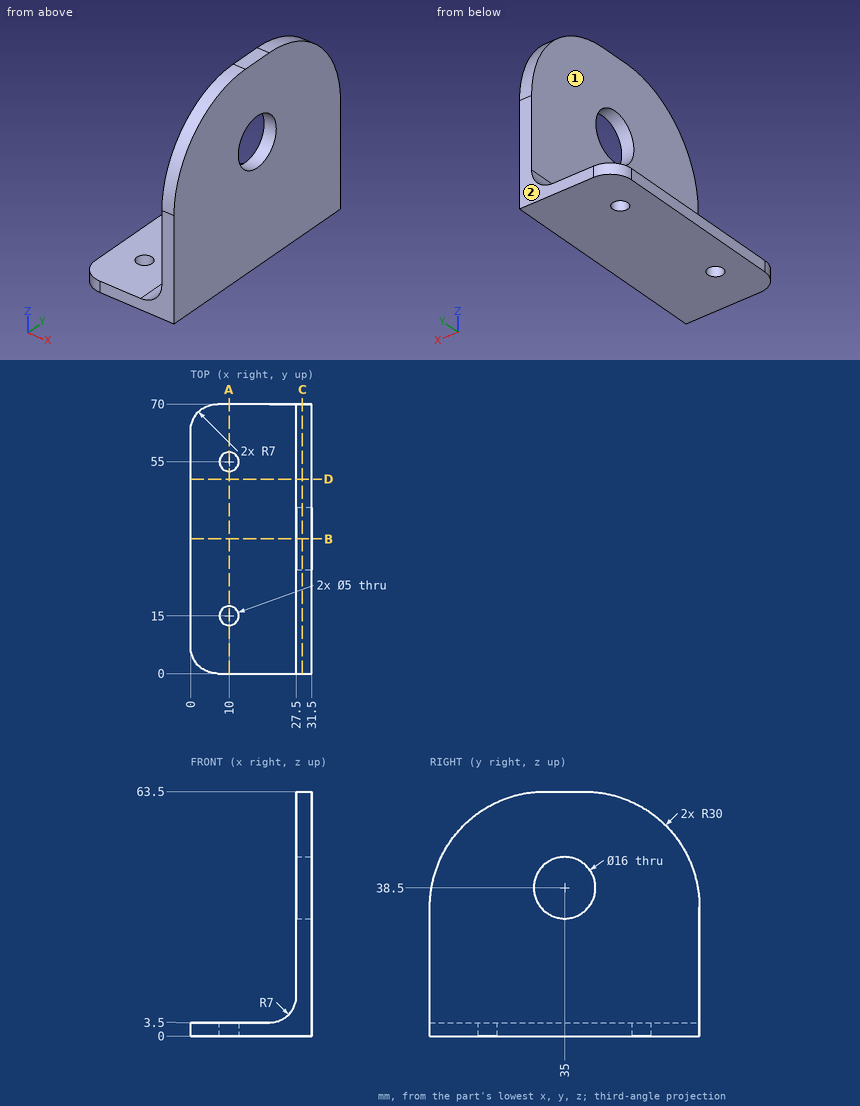
Verification items for this drawing (mm, ordinates from the low corner). A direction names the side the tool comes from. Give positions to 0.01 mm unless a question says otherwise; leave off trailing zeros. Write each loop counter-clockwise with the first axis right and the second up, starting at its lowest first coordinate (ties: lowest second). Pieces come first, ordered by that corner, then holes. Notation, with made-up numbers: (21.25, 46.5) - (35.25, 46.5) arc R20 ccw to (35.25, 76.5) - close; hole circle Ø6 at (67.25, 39). An arc over 180 degrees is marked (long way). Answer as CSV lines item,"result". Start each with the question number.
1. Sectioned sample at C-C (x = 29). Record the boundary of the cut face in (y, z), then the cut area to 3 significant figures.
2. Set-up check for the marked faces 1 and 2: record each of +Z, -Z, +X, -X, +Y, -Y from which the full face is reachable in a straight line by a thin tool's end or side.
3. Thickness scan on line 1 (Y direction, x = 10, z = 1.55); line 2 (Z direction, x = 30, y = 35); line 3 (Z direction, x = 17.5, y = 21.5). Record the ranges inside material, lowest first.
4. Sectioned sample at A-A (x = 10). Record the boundary of the cut face in (y, z), then the cut area to 3 significant figures.
5. Sectioned sample at D-D (y = 50.5). Record the boundary of the cut face in (x, z).
6. Sectioned sample at B-B (y = 35). Record the boundary of the cut face in (x, z), then the cut area to 3 significant figures.
7. Depth check by flat-ended pin: pin 1 (12 mm diameter, centred on x = 8.5, y = 41, fed in from +Z); pin 2 (1.5 mm diameter, centred on x = 27, z = 50, fed in from +Y); pin 3 (16.5 mm diameter, centred on x = 13.5, y = 23, fed in from +Z). Enter the tip coordinate at first touch or a pass-through.
Derived:
1,outline,"(0, 0) - (70, 0) - (70, 33.5) arc R30 ccw to (40, 63.5) - (30, 63.5) arc R30 ccw to (0, 33.5) - close; hole circle Ø16 at (35, 38.5)"
1,area,"3,860 mm²"
2,face 1,"+Z, -X, +Y, -Y"
2,face 2,"+Z, -Z, +X, -X, +Y"
3,line 1,"0 to 12.5, 17.5 to 52.5, 57.5 to 70"
3,line 2,"0 to 30.5, 46.5 to 63.5"
3,line 3,"0 to 3.5"
4,outline,"(0, 0) - (12.5, 0) - (12.5, 3.5) - (0, 3.5) - close; (17.5, 0) - (52.5, 0) - (52.5, 3.5) - (17.5, 3.5) - close; (57.5, 0) - (70, 0) - (70, 3.5) - (57.5, 3.5) - close"
4,area,"210 mm²"
5,outline,"(0, 0) - (31.5, 0) - (31.5, 61.6) - (27.5, 61.6) - (27.5, 10.5) arc R7 cw to (20.5, 3.5) - (0, 3.5) - close"
6,outline,"(0, 0) - (31.5, 0) - (31.5, 30.5) - (27.5, 30.5) - (27.5, 10.5) arc R7 cw to (20.5, 3.5) - (0, 3.5) - close; (27.5, 46.5) - (31.5, 46.5) - (31.5, 63.5) - (27.5, 63.5) - close"
6,area,"297 mm²"
7,pin 1,"z = 3.5"
7,pin 2,"y = 65.41"
7,pin 3,"z = 3.61"
